Autodesk Inventor part; units mm, degrees
ref_plane "YZ Plane" through (0, 0, 0) normal (1, 0, 0) x (0, 1, 0)
ref_plane "XZ Plane" through (0, 0, 0) normal (0, 1, 0) x (-1, 0, 0)
ref_plane "XY Plane" through (0, 0, 0) normal (0, 0, 1) x (1, 0, 0)
sketch "Sketch1" plane through (0, 0, 0) normal (0, 0, 1) x (1, 0, 0)
  line L0 (-6.5, 4.5) -> (6.5, 4.5)
  line L1 (6.5, 4.5) -> (6.5, -4.5)
  line L2 (6.5, -4.5) -> (-6.5, -4.5)
  line L3 (-6.5, -4.5) -> (-6.5, 4.5)
  point P0 (0, 0)
  dimension "d0" = 13
  dimension "d1" = 9
  dimension "d2" = 4.5
  dimension "d3" = 6.5
extrude "Extrusion1" add sketch "Sketch1" along normal blind 7
sketch "Sketch2" plane through (-6.5, -4.5, 0) normal (0, -1, 0) x (1, 0, 0)
  line L0 (1, 4.5) -> (1.5, 4.5)
  line L1 (1.5, 4.5) -> (1.5, 2.5)
  line L2 (1.5, 2.5) -> (1, 2.5)
  line L3 (1, 2.5) -> (1, 4.5)
  line L4 (11.5, 4.5) -> (12, 4.5)
  line L5 (12, 4.5) -> (12, 2.5)
  line L6 (12, 2.5) -> (11.5, 2.5)
  line L7 (11.5, 2.5) -> (11.5, 4.5)
  line L8 (6.25, 2.5) -> (6.75, 2.5)
  line L9 (6.75, 2.5) -> (6.75, 4.5)
  line L10 (6.75, 4.5) -> (6.25, 4.5)
  line L11 (6.25, 4.5) -> (6.25, 2.5)
  line L12 (0, 0) -> (0, 7)
  line L13 (13, 0) -> (13, 7)
  line L14 (0, 7) -> (13, 7)
  point P0 (6.5, 0)
  dimension "d6" = 0.5
  dimension "d7" = 0.5
  dimension "d8" = 0.5
  dimension "d9" = 1
  dimension "d10" = 1
  dimension "d11" = 6.25
  dimension "d12" = 6.25
  dimension "d13" = 2
  dimension "d14" = 2
  dimension "d15" = 2
  dimension "d16" = 2.5
extrude "Extrusion2" add sketch "Sketch2" along normal blind 4
sketch "Sketch3" plane through (-6.5, 4.5, 0) normal (0, 1, 0) x (1, 0, 0)
  line L0 (0, -7) -> (13, -7)
  line L1 (0, 0) -> (0, -7)
  circle A0 centre (6.5, -3.5) radius 2.65
  point P0 (6.5, 0)
  point P1 (6.5, -7)
  point P2 (0, -3.5)
  dimension "d19" = 5.3
extrude "Extrusion3" add sketch "Sketch3" along normal blind 9
sketch "Sketch4" plane through (0, 13.5, 3.5) normal (0, 1, 0) x (1, 0, 0)
  line L0 (-0.5, 0) -> (0.5, 0)
  line L1 (0.5, 0) -> (0.5, 0.1)
  line L2 (0.5, 0.1) -> (-0.5, 0.1)
  line L3 (-0.5, 0.1) -> (-0.5, 0)
  circle A0 centre (0, 0) radius 2.65
  point P0 (0, 3.5)
  dimension "d22" = 0
  dimension "d23" = 0.1
  dimension "d24" = 0.5
  dimension "d25" = 0.5
extrude "Extrusion4" add sketch "Sketch4" along normal blind 3 contours L3 L2 L1 L0
sketch "Sketch5" plane through (-0.5, 13.5, 3.5) normal (0, 0, 1) x (1, 0, 0)
  line L0 (3.15, 0) -> (-2.15, 0)
  line L1 (0, 0) -> (0, 3)
  line L2 (1.1, 0) -> (2, 9)
  arc A0 (2, 9) -> (0.5, 10) centre (0.5167, 8.4001) ccw
  line L3 (0.5, 10) -> (0.5, 0)
  line L4 (1.1, 0) -> (0.5, 0)
  line L5 (0.5, -28.4463) -> (0.5, 16.6776)
  point P0 (0.5, -13.5)
  point P1 (2, 10)
  dimension "d28" = 10
  dimension "d29" = 1.5
  dimension "d30" = 1.1
  dimension "d31" = 1
  dimension "d32" = 1.6
revolve "Revolution1" add sketch "Sketch5" angle 360 about axis through (0, -10, 3.5) along (0, 1, 0)
thread "Thread1"
properties part number "switch-mockup"
Model file for the job. Use its own axes, mm. A direction names the side the tool comes from. Coordinates: 2 decimals unless noted, no trailing zeros. Write each loop counter-clockwise with the first axis right and the second up, starting at its lowest first coordinate (ties: lowest second). Pieces come first, ordered by that corner, then holes. Notation, with made-up numbers: (-20.75, -31) -> (35.25, -31) arc R29 ccw to (35.25, -7) -> close; hole circle Ø4 at (9.25, 13). An arc over 180 degrees is marked (long way). One line per item, written item: value. Start each with the question number.
1) Which spindle directions (+Z, -Z, +X, -X, +Y, -Y) get a long thin tool onto all of the face, cutting with end or side? Do faces 1 (the face through (5, -6, 3)), 2 (the face through (6.5, 0, 3)), 3 (the face through (5.5, -6, 4)), 4 (the face through (-0.138, 18.063, 2.453)). Say none if no direction does.
2) Probe probe 1 along X at (y, z) = (9, 3.5); probe 2 along Y at (x, z) = (2.5, 5.5); probe 3 along Y at (x, z) = (-1, 1.5). List the from-to ranges inside material, lowest first.
3) Flat gauge pins, fed straight in: pin 1 Ø1 at (y, z) = (-6, 3.5) entering from +X; pin 2 Ø2 at (y, z) = (-7, 3.5) entering from -X; pin 3 Ø2 at (x, z) = (-3, 2) entering from +Y. Where does each tip first touch, or does it go through?
4) Pull direction X, two halves, no side cores. Call faces 5 (the face through (-0.57, 8.94, 0.91)), 6 (the face through (-5.5, -6, 3)), 7 (the face through (2, -4.5, 3)): +X half, -X half, draft (parallel to the pull), parting line (faces both ways), or undercut.
5) Slice it at C-C on y = 20. Write the cut outline in (x, z).
6) Slice it at B-B on y = 5. Write the cut outline in (x, z), then the cut area to 3 significant figures.
7) Slice it at A-A on z = 5.75. Write the cut outline in (x, y).
Answers follow:
1. face 1: +Z, -Z, -Y
1. face 2: +Z, -Z, +X, +Y, -Y
1. face 3: +Z, -Z, +X, -Y
1. face 4: none
2. probe 1: -2.65 to 2.65
2. probe 2: -4.5 to 4.5
2. probe 3: -4.5 to 13.5
3. pin 1: x = 5.5
3. pin 2: x = -5.5
3. pin 3: y = 13.5
4. face 5: parting line
4. face 6: -X half
4. face 7: undercut
5. outline: circle Ø2.5 at (0, 3.5)
6. outline: circle Ø5.3 at (0, 3.5)
6. area: 22.1 mm2
7. outline: (-6.5, -4.5) -> (6.5, -4.5) -> (6.5, 4.5) -> (1.4, 4.5) -> (1.4, 13.5) -> (-1.4, 13.5) -> (-1.4, 4.5) -> (-6.5, 4.5) -> close
